Can you work these out from the model? Positions are in its coordinate system, mm. A direction names the side the tool comes from. Give positions to 0.01 mm unless a question says otherwise; leave off trailing zeros. Loops run counter-clockwise (first coordinate to the right, second up) from the corner with the lowest first, then second, coordinate; pieces in that order, holes last.
from build123d import *

# Parameters (mm, degrees)
F1_DEPTH = 63.5
F0_W     = 25.4
F0_H     = 10.2552045137
F2_DEPTH = 25.4
F3_DEPTH = 7.9375


with BuildPart() as f1:
    # F0 (on Front) → F1 (new body, symmetric)
    with BuildSketch(Plane.XZ):
        Polygon((-41.275, 9.525), (-41.275, -9.525), (41.275, -9.525), (41.275, 9.525), (31.0197954863, 9.525), align=None)
    extrude(amount=F1_DEPTH, both=True)

    # F0 (on Front) → F2 (join, symmetric)
    with BuildSketch(Plane.XZ):
        with BuildLine():
            Line((31.0197954863, 9.525), (41.275, 9.525))
            Line((41.275, 9.525), (41.275, 27.0218505154))
            ThreePointArc((41.275, 27.0218505154), (46.2216382961, 38.5364731957), (57.978815492, 42.8752))
            Line((57.978815492, 42.8752), (60.325, 42.8752))
            Line((60.325, 42.8752), (60.325, 53.1304045137))
            Line((60.325, 53.1304045137), (58.2134829791, 53.1304045137))
            add(Edge.make_bspline(
                [(55.9138915665, 53.1228011469), (56.6888329701, 53.1264926522), (57.455577593, 53.128923314), (58.2134829791, 53.1304045137)],
                knots=[106.4066342926, 106.4066342926, 106.4066342926, 106.4066342926, 108.6249950439, 108.6249950439, 108.6249950439, 108.6249950439], degree=3))
            ThreePointArc((55.9138915665, 53.1228011469), (38.2411746254, 45.0563704946), (31.0197954863, 27.0218505154))
            Line((31.0197954863, 27.0218505154), (31.0197954863, 9.525))
        make_face()
        with Locations((73.025, 48.0028022568)):
            Rectangle(F0_W, F0_H)
    extrude(amount=F2_DEPTH, both=True)

    # F0 (on Front) → F3 (join, symmetric)
    with BuildSketch(Plane.XZ):
        with BuildLine():
            add(Edge.make_bspline(
                [(-41.275, 9.525), (-37.2872071441, 49.8677554135), (18.7427928229, 52.94573317), (55.9138915665, 53.1228011469)],
                knots=[0, 0, 0, 0, 106.4066342926, 106.4066342926, 106.4066342926, 106.4066342926], degree=3))
            Line((-41.275, 9.525), (31.0197954863, 9.525))
            Line((31.0197954863, 9.525), (31.0197954863, 27.0218505154))
            ThreePointArc((31.0197954863, 27.0218505154), (38.2411746254, 45.0563704946), (55.9138915665, 53.1228011469))
        make_face()
    extrude(amount=F3_DEPTH, both=True)

    # F0 (on Front) → F4 (revolve)
    with BuildSketch(Plane.XZ):
        Polygon((85.725, 66.675), (85.725, 53.1304045137), (85.725, 42.8752), (85.725, 38.1), (111.125, 38.1), (111.125, 66.675), align=None)
    revolve(axis=Axis((85.725, 0, 52.3875), (0, 0, -1)))


solid = f1.part
(1) Thinking about a two-plate mould opening in X: for faces 5 (the flat face through (31.02, 17, 18)), 6 (the flat face through (1, 35, 9.525)), 7 (the cylindrical face through (46.09, -0.36, 38.41)), which applies, pulls with the +X half, pulls with the -X half, needs draft (parallel to the pull), parting line crosses it, or undercut?
Returned:
face 5: pulls with the -X half
face 6: needs draft
face 7: undercut
(2) Suppose I cut it at A-A on z = 7.5. List the corners of the cut face in (x, y) for me (3 decimals), plus the area to 3 significant figures.
Returned:
outline: (-41.275, -63.5) - (41.275, -63.5) - (41.275, 63.5) - (-41.275, 63.5) - close
area: 10,500 mm2
(3) Which directions (+Z, -Z, +X, -X, +Y, -Y) give clear straight access to the entire face, cutting with the end or side of a thin tool? Please do faces 1 (the flat face through (31.02, -17, 18)), 2 (the flat face through (-3, 7.938, 27)), 3 (the flat face through (48, -25.4, 41)), 4 (the flat face through (48, 25.4, 41)).
Returned:
face 1: +Z, -X, -Y
face 2: +Z, -X, +Y
face 3: +Z, +X, -X, -Y
face 4: +Z, +X, -X, +Y
(4) Will these pins go through, and if not, where does the flat tip stop? P1, Ø22, axis at x = 9, z = 40, coming from the -Y side; P2, Ø6, axis at y = -16, z = 11.5, coming from the +X side (3 decimals); P3, Ø22, axis at x = 71.5, y = -0.5, coming from the -Z side; P4, Ø3, axis at y = 1, z = 39, coming from the +X side (3 decimals).
Returned:
P1: stops at y = -7.94
P2: stops at x = 41.275
P3: stops at z = 38.1
P4: stops at x = 111.125
(5) Suppose I cut it at B-B on y = 47. List the corners of the cut face in (x, z) for me (3 decimals).
Returned:
outline: (-41.275, -9.525) - (41.275, -9.525) - (41.275, 9.525) - (-41.275, 9.525) - close
(6) Suppose I cut it at C-C on x = 82.5. List the corners of the cut face in (y, z) for me (3 decimals), plus the area to 3 significant figures.
Returned:
outline: (-25.4, 42.875) - (-25.194, 42.875) - (-25.194, 38.1) - (25.194, 38.1) - (25.194, 42.875) - (25.4, 42.875) - (25.4, 53.13) - (25.194, 53.13) - (25.194, 66.675) - (-25.194, 66.675) - (-25.194, 53.13) - (-25.4, 53.13) - close
area: 1,440 mm2
(7) Please list where these lines run through material, in increasing order: probe 1 along Z at (x, y) = (-11, -54) (3 decimals); probe 2 along Y at (x, z) = (71.5, 48); probe 3 along Z at (x, y) = (62, 3.5) (3 decimals).
Returned:
probe 1: z = -9.525 to 9.525
probe 2: y = -25.4 to 25.4
probe 3: z = 38.1 to 66.675
